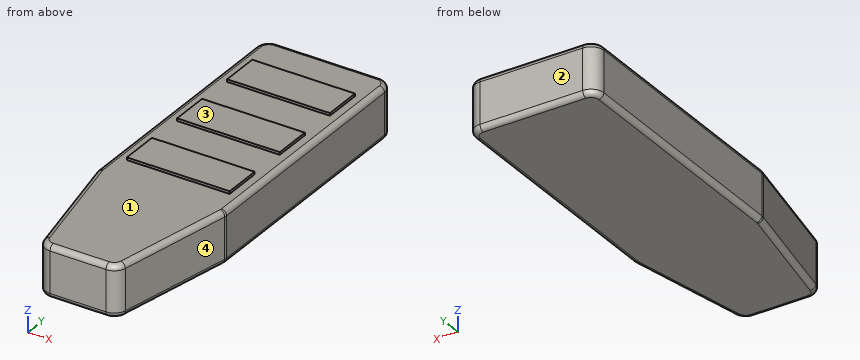
from build123d import *

# Parameters (mm, degrees)
F1_DEPTH = 20
F2_R     = 2
F3_W     = 40
F3_H     = 15
F4_DEPTH = 1


with BuildPart() as f1:
    # F0 (on Top) → F1 (new body)
    with BuildSketch(Plane.XY):
        with BuildLine():
            Line((20, 75), (-20, 75))
            ThreePointArc((-20, 75), (-23.535534, 73.535534), (-25, 70))
            Line((-25, 70), (-25, -24.504902))
            ThreePointArc((-25, -24.504902), (-24.975667, -24.997591), (-24.902903, -25.485483))
            Line((-24.902903, -25.485483), (-15.803884, -70.980581))
            ThreePointArc((-15.803884, -70.980581), (-14.070925, -73.866711), (-10.90098, -75))
            Line((-10.90098, -75), (10.90098, -75))
            ThreePointArc((10.90098, -75), (14.070925, -73.866711), (15.803884, -70.980581))
            Line((15.803884, -70.980581), (24.902903, -25.485483))
            ThreePointArc((24.902903, -25.485483), (24.975667, -24.997591), (25, -24.504902))
            Line((25, -24.504902), (25, 70))
            ThreePointArc((25, 70), (23.535534, 73.535534), (20, 75))
        make_face()
    extrude(amount=F1_DEPTH)

    # F2
    f2_edges = [f1.edges().sort_by_distance(p)[0] for p in [
        (-25, 22.747549, 20),
        (-20.353394, -48.233032, 0),
    ]]
    fillet(f2_edges, radius=F2_R)

    # F3 (on face) → F4 (join)
    with BuildSketch(Plane.XY.offset(20)):
        with Locations((0, 52.5)):
            Rectangle(F3_W, F3_H)
        with Locations((0, 22.5)):
            Rectangle(F3_W, F3_H)
        with Locations((0, -7.5)):
            Rectangle(F3_W, F3_H)
    extrude(amount=F4_DEPTH)


solid = f1.part
Source: CAD feature listing. Evaluate the final solid. Frame: model axes, mm. Face numbers are marked on the shaded views. Coordinates: 2 decimals unless noted, no trailing zeros. Order: outer loops, then holes, each group sorted by start corner. A loop starts at its lowest first (then second) coordinate and runs counter-clockwise, first axis right, second up. Notation, with made-up numbers: M -5,43 L 18,43 A20 cw 18,65 Z; hole C -24,-3.5 d4. An arc over 180 degrees is marked long. Write each question's results on one line, items separated by ' | '. Start each with the question number.
Item 1: Line query: probe 1 along Z at (x, y) = (-18.5, 35.5); probe 2 along Y at (x, z) = (-11, 10.5); probe 3 along X at (y, z) = (-46.5, 8.75). Output: solid intervals per line, ascending.
Item 2: Cut plane A-A (y = 65.5). Return loops of the section in (x, z).
Item 3: Draft query along Y for the marked faces 1, 2, 3 and 4. Return one class per face: pulls with the +Y half, pulls with the -Y half, needs draft (parallel to the pull), parting line crosses it, or undercut.
Item 4: Cut plane C-C (x = 0.5). Return loops of the section in (y, z), and give its area (3 significant figures).
Item 5: Cut plane B-B (z = 6.25). Return loops of the section in (x, y).
Item 6: First-contact query: pin 1 Ø12 at (y, z) = (-59, 10) entering from -X; pin 2 Ø0.8 at (y, z) = (21.5, 20.5) entering from -X; pin 3 Ø0.8 at (x, z) = (-5, 20.5) entering from +Y. Flat tips, straight axial feed; report the tip coordinate or a pass-through.
Checked values:
1) probe 1: z = 0 to 20 | probe 2: y = -75 to 75 | probe 3: x = -20.7 to 20.7
2) outline: M -25,2 A2 ccw -23,0 L 23,0 A2 ccw 25,2 L 25,18 A2 ccw 23,20 L -23,20 A2 ccw -25,18 Z
3) face 1: undercut | face 2: pulls with the +Y half | face 3: needs draft | face 4: pulls with the -Y half
4) outline: M -75,2 A2 ccw -73,0 L 73,0 A2 ccw 75,2 L 75,18 A2 ccw 73,20 L 60,20 L 60,21 L 45,21 L 45,20 L 30,20 L 30,21 L 15,21 L 15,20 L 0,20 L 0,21 L -15,21 L -15,20 L -73,20 A2 ccw -75,18 Z | area: 3,040 mm2
5) outline: M -25,-24.5 A5 ccw -24.9,-25.49 L -15.8,-70.98 A5 ccw -10.9,-75 L 10.9,-75 A5 ccw 15.8,-70.98 L 24.9,-25.49 A5 ccw 25,-24.5 L 25,70 A5 ccw 20,75 L -20,75 A5 ccw -25,70 Z
6) pin 1: stops at x = -19.4 | pin 2: stops at x = -20 | pin 3: stops at y = 60
